from build123d import *

# Parameters (mm, degrees)
F1_DEPTH = 5
F2_R     = 2


with BuildPart() as f1:
    # F0 (on Front) → F1 (new body)
    with BuildSketch(Plane.XZ):
        Polygon((0, -33), (0, 0), (-27.65, 0), (-27.65, -28), (-30.95, -28), (-30.95, 0), (-37.6, 0), (-37.6, -33), align=None)
    extrude(amount=-F1_DEPTH)

    # F2
    f2_edges = [f1.edges().sort_by_distance(p)[0] for p in [
        (-37.6, 2.5, 0),
        (-30.95, 2.5, 0),
        (-27.65, 2.5, 0),
        (0, 2.5, 0),
        (0, 2.5, -33),
        (-37.6, 2.5, -33),
    ]]
    fillet(f2_edges, radius=F2_R)


solid = f1.part
Here's how the part is built. I have some questions about the finished solid (model axes, mm). A direction names the side the tool comes from. Round coordinates to 2 decimals unless told otherwise and drop trailing zeros. Order: outer loops, then holes, each group sorted by start corner. A loop starts at its lowest first (then second) coordinate and runs counter-clockwise, first axis right, second up. Notation, with made-up numbers: (44, 33) -> (93, 33) arc R17 cw to (93, 66) -> close; hole circle Ø4 at (73.5, 80). An arc over 180 degrees is marked (long way). Return JSON: item names as keys, results as strings.
Q1. If we section it at B-B on y = 2.95: List the corners of the cut face in (x, z) for me.
Filled sheet:
{"outline": "(-37.6, -31) arc R2 ccw to (-35.6, -33) -> (-2, -33) arc R2 ccw to (0, -31) -> (0, -2) arc R2 ccw to (-2, 0) -> (-25.65, 0) arc R2 ccw to (-27.65, -2) -> (-27.65, -28) -> (-30.95, -28) -> (-30.95, -2) arc R2 ccw to (-32.95, 0) -> (-35.6, 0) arc R2 ccw to (-37.6, -2) -> close"}
Q2. If we section it at C-C on x = -27: List the corners of the cut face in (y, z) for me.
Filled sheet:
{"outline": "(0, -33) -> (5, -33) -> (5, -0.52) -> (0, -0.52) -> close"}
Q3. I need wall thicknesses on line 1 along X through (y, z) = (3.85, -6.5). Which ranges of the line are inside material? Lowest first, please. Write a range as from..to.
Filled sheet:
{"line 1": "x = -37.6..-30.95, -27.65..0"}
Q4. If we mould it in two halves opening along X, with no side actions, what happens to faces 1 (the flat face through (-19, 5, -16)), 2 (the flat face through (-29, 2, -28)), 3 (the cylindrical face through (-37, 2.54, -0.57)), 4 (the cylindrical face through (-0.57, 2.54, -32.4))? For each: released by +X, released by -X, zero draft, split by the parting line, or undercut.
Filled sheet:
{"face 1": "zero draft", "face 2": "undercut", "face 3": "released by -X", "face 4": "released by +X"}
Q5. If we section it at A-A on z = -14: List the corners of the cut face in (x, y) for me.
Filled sheet:
{"outline": "(-37.6, 0) -> (-30.95, 0) -> (-30.95, 5) -> (-37.6, 5) -> close; (-27.65, 0) -> (0, 0) -> (0, 5) -> (-27.65, 5) -> close"}
Q6. Which directions (+Z, -Z, +X, -X, +Y, -Y) give clear straight access to the entire face, cutting with the end or side of a thin tool? Please do faces 5 (the flat face through (-30.95, 2, -15)), 6 (the flat face through (-34, 2, 0)).
Filled sheet:
{"face 5": "+Z, +Y, -Y", "face 6": "+Z, +X, -X, +Y, -Y"}
